Input: dimensioned drawing with shaded views. Units: mm. Origin: part minimum x, y, z. Coordinates: 2 decimals unless noted, no trailing zeros. Loops run counter-clockwise (first coordinate to the right, second up) from the corner with the lowest first, then second, coordinate; pieces in that order, holes last.
Item 1: Contact query for a flat-ended pin moving along its axis: P1, Ø2.5, axis at x = 15, z = 91, coming from the -Y side. Output: stop coordinate, or through.
Item 2: Section A-A on z = 46. Return loops of the section in (x, y).
Item 3: Section B-B on x = 106. Return loops of the section in (y, z), and give its area (4 significant figures).
Item 4: Ray query, line 1 along Z through (x, y) = (38.5, 0.4); line 2 along X through (y, z) = (0.15, 17); line 3 along Z through (x, y) = (100, 0.7). Return the intervals inside material, ascending.
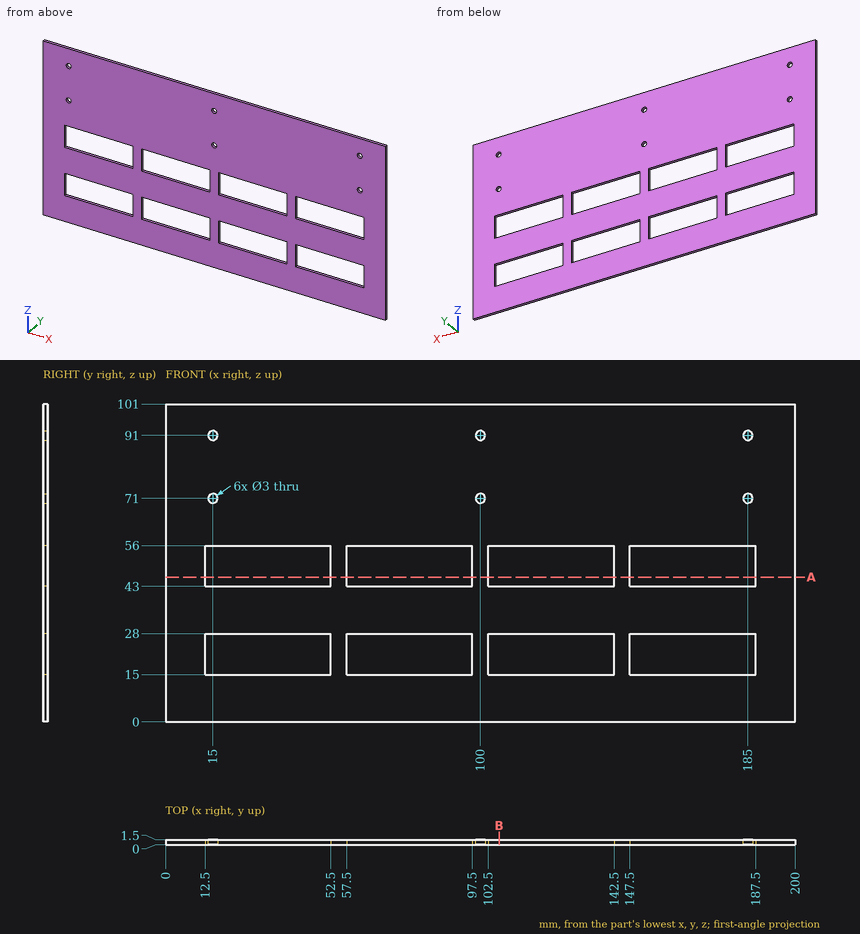
Results found:
1. P1: passes through
2. outline: (0, 0) - (12.5, 0) - (12.5, 1.5) - (0, 1.5) - close; (52.5, 0) - (57.5, 0) - (57.5, 1.5) - (52.5, 1.5) - close; (97.5, 0) - (102.5, 0) - (102.5, 1.5) - (97.5, 1.5) - close; (142.5, 0) - (147.5, 0) - (147.5, 1.5) - (142.5, 1.5) - close; (187.5, 0) - (200, 0) - (200, 1.5) - (187.5, 1.5) - close
3. outline: (0, 0) - (1.5, 0) - (1.5, 15) - (0, 15) - close; (0, 28) - (1.5, 28) - (1.5, 43) - (0, 43) - close; (0, 56) - (1.5, 56) - (1.5, 101) - (0, 101) - close
3. area: 112.5 mm2
4. line 1: z = 0 to 15, 28 to 43, 56 to 101
4. line 2: x = 0 to 12.5, 52.5 to 57.5, 97.5 to 102.5, 142.5 to 147.5, 187.5 to 200
4. line 3: z = 0 to 69.5, 72.5 to 89.5, 92.5 to 101
